Geometry: final body of the model. Coordinates: model frame, mm. A direction names the side the tool comes from. Give positions to 0.01 mm unless a question says otherwise; leave off trailing zeros. Loops run counter-clockwise (first coordinate to the right, second up) from the corner with the lowest first, then second, coordinate; pieces in that order, holes last.
1. Material intervals for line 1 along X through (y, z) = (-27, -23); line 2 along X through (y, z) = (-16, 44.5); line 3 along Z through (x, y) = (-41, -89.5), sorted ascending.
2. Access query for faces 1 (the face through (-59.589, -49, -1)), 2 (the face through (27.356, -49, 46)), 3 (the face through (-4.806, -9.427, -38.905)). Directions: +Z, -Z, +X, -X, +Y, -Y. A direction counts if a zero-diameter tool reaches every point of the face in a straight line with its end or side. Return the directions, or none.
3. Section C-C, the plane y = -40.5. Output: boundary loops of the cut face in (x, z).
4. Draft query along Y for faces 4 (the face through (1.326, -47, -39)), 5 (the face through (-37.644, -49, 46)), 6 (the face through (0, -100, -35)). Return one class per face: +Y half, -Y half, draft (parallel to the pull), parting line (faces both ways), or undercut.
5. Section A-A, the plane x = -43.5. Output: boundary loops of the cut face in (y, z).
6. First-contact query: P1, Ø10, axis at x = -16.5, y = -52, coming from the +Z side; P2, Ø10.5, axis at y = -54, z = -39.5, coming from the -X side; P3, Ø1, axis at y = -88.5, z = -15.5, coming from the +X side. Flat tips, straight axial feed; report the tip coordinate or a pass-through.
7. Section B-B, the plane z = -10. Output: boundary loops of the cut face in (x, y), then the cut area to 3 significant figures.
from build123d import *

# Parameters (mm, degrees)
F1_DEPTH = 100
F3_DEPTH = 29


with BuildPart() as f1:
    # F0 (on Front) → F1 (new body)
    with BuildSketch(Plane.XZ):
        Polygon((-59.58884, 51.302213), (-72.644392, 51.302213), (-72.644392, 41.302213), (-59.58884, 41.302213), (-59.58884, -33.975578), (-59.58884, -43.697798), (-49.58884, -43.697798), (40.41116, -43.697798), (50.41116, -43.697798), (50.41116, -33.975578), (50.41116, 41.302213), (62.355608, 41.302213), (62.355608, 51.302213), (50.41116, 51.302213), (40.41116, 51.302213), (27.355608, 51.302213), (27.355608, 41.302213), (40.41116, 41.302213), (40.41116, -33.975578), (-49.58884, -33.975578), (-49.58884, 41.302213), (-37.644392, 41.302213), (-37.644392, 51.302213), (-49.58884, 51.302213), align=None)
    extrude(amount=F1_DEPTH)

    # F2 (on face) → F3 (cut)
    with BuildSketch(Plane(origin=(0, 0, -43.697798), x_dir=(1, 0, 0), z_dir=(0, 0, -1))):
        with BuildLine():
            ThreePointArc((1.325937, 80.42562), (-4.674063, 86.42562), (-10.674063, 80.42562))
            Line((-10.674063, 80.42562), (-10.674063, 15.42562))
            ThreePointArc((-10.674063, 15.42562), (-4.674063, 9.42562), (1.325937, 15.42562))
            Line((1.325937, 15.42562), (1.325937, 80.42562))
        make_face()
    extrude(amount=-F3_DEPTH, mode=Mode.SUBTRACT)


solid = f1.part
Answers below:
1. line 1: x = -59.59 to -49.59, 40.41 to 50.41
1. line 2: x = -72.64 to -37.64, 27.36 to 62.36
1. line 3: z = -43.7 to -33.98, 41.3 to 51.3
2. face 1: -Z, -X, +Y, -Y
2. face 2: +Z, +Y, -Y
2. face 3: +Z, -Z
3. outline: (-72.64, 41.3) - (-59.59, 41.3) - (-59.59, -43.7) - (-10.67, -43.7) - (-10.67, -33.98) - (-49.59, -33.98) - (-49.59, 41.3) - (-37.64, 41.3) - (-37.64, 51.3) - (-72.64, 51.3) - close; (1.33, -43.7) - (50.41, -43.7) - (50.41, 41.3) - (62.36, 41.3) - (62.36, 51.3) - (27.36, 51.3) - (27.36, 41.3) - (40.41, 41.3) - (40.41, -33.98) - (1.33, -33.98) - close
4. face 4: undercut
4. face 5: draft
4. face 6: -Y half
5. outline: (-100, -43.7) - (0, -43.7) - (0, -33.98) - (-100, -33.98) - close; (-100, 41.3) - (0, 41.3) - (0, 51.3) - (-100, 51.3) - close
6. P1: stops at z = -33.98
6. P2: stops at x = -59.59
6. P3: stops at x = 50.41
7. outline: (-59.59, -100) - (-49.59, -100) - (-49.59, 0) - (-59.59, 0) - close; (40.41, -100) - (50.41, -100) - (50.41, 0) - (40.41, 0) - close
7. area: 2,000 mm2
